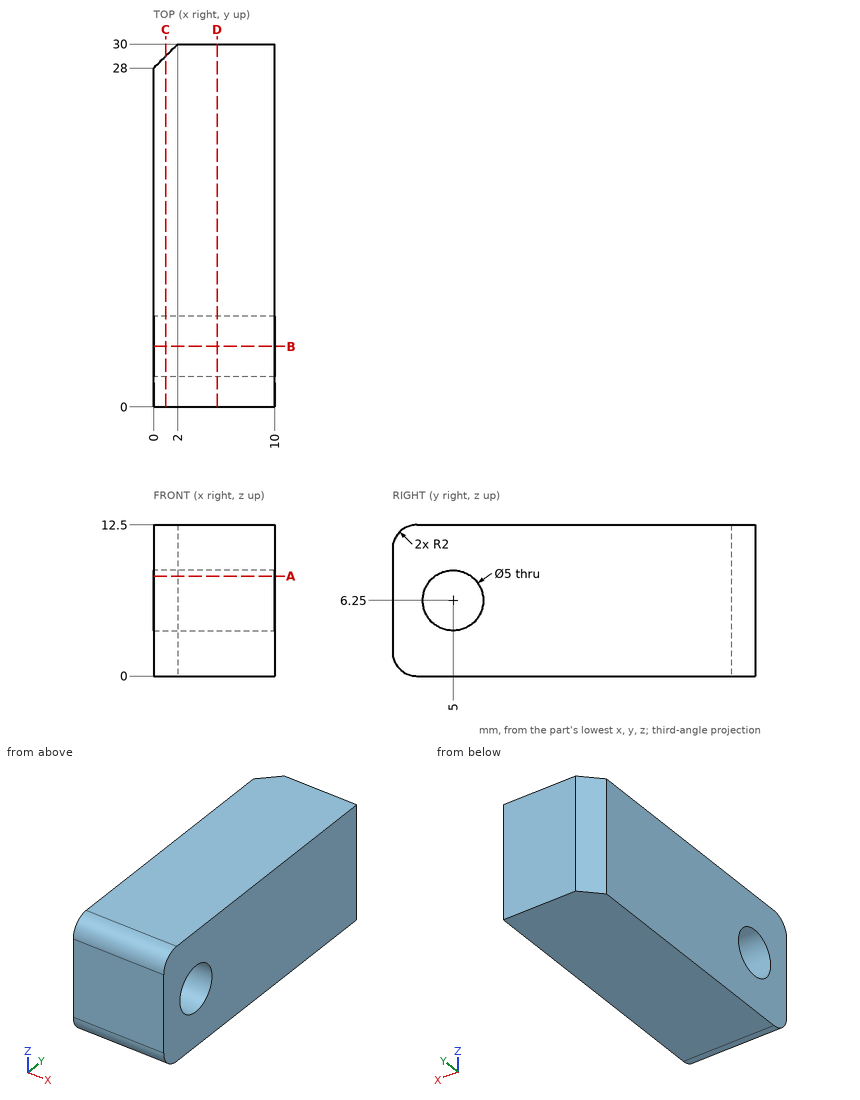
Job drawing, mm, ordinate dimensions from the low corner. One solid piece. Give positions to 0.01 mm unless a question says otherwise; leave off trailing zeros. Order: outer loops, then holes, each group sorted by start corner. A loop starts at its lowest first (then second) coordinate and runs counter-clockwise, first axis right, second up. Notation, with made-up numbers: M -3,-1 L 3,-1 A20 cw 3,17 Z; hole C -4.75,59.25 d7. An arc over 180 degrees is marked long. Put each result on its own line as item: value. Start each with the question number.
(1) Band-saw the part on B-B on y = 5. Give the cut face in (x, z).
(2) Band-saw the part on D-D on x = 5.25. Give the cut face in (y, z).
(3) Band-saw the part on C-C on x = 1. Give the cut face in (y, z), then the cut area to 3 significant figures.
(4) Band-saw the part on A-A on z = 8.25. Give the cut face in (x, y), then the cut area to 3 significant figures.
(5) Drill centre lines: L1, parallel to Y at x = 2.5, z = 6.25; L2, parallel to Z at x = 3.75, y = 5; L3, parallel to Y at x = 5.25, z = 4.5. Where is each one in solid material? Low to high. Write a range as [from, to].
Results below:
1. outline: M 0,0 L 10,0 L 10,3.75 L 0,3.75 Z; M 0,8.75 L 10,8.75 L 10,12.5 L 0,12.5 Z
2. outline: M 0,2 A2 ccw 2,0 L 30,0 L 30,12.5 L 2,12.5 A2 ccw 0,10.5 Z; hole C 5,6.25 d5
3. outline: M 0,2 A2 ccw 2,0 L 29,0 L 29,12.5 L 2,12.5 A2 ccw 0,10.5 Z; hole C 5,6.25 d5
3. area: 341 mm2
4. outline: M 0,0 L 10,0 L 10,3.5 L 0,3.5 Z; M 0,6.5 L 10,6.5 L 10,30 L 2,30 L 0,28 Z
4. area: 268 mm2
5. L1: y = [0, 2.5], [7.5, 30]
5. L2: z = [0, 3.75], [8.75, 12.5]
5. L3: y = [0, 3.21], [6.79, 30]
